from build123d import *

# Parameters (mm, degrees)
F0_W     = 36
F0_H     = 36
F1_DEPTH = 243
F3_DEPTH = 40.001


# Not quite as in the source:
# - a pattern or mirror of a feature is missing from the dataset's text; its kind, count and spacing are read off the source's solid


with BuildPart() as f1:
    # F0 (on Top) → F1 (new body, symmetric)
    with BuildSketch(Plane.XY):
        with BuildLine():
            Line((17, 20), (-17, 20))
            ThreePointArc((-17, 20), (-19.1213203436, 19.1213203436), (-20, 17))
            Line((-20, 17), (-20, -17))
            ThreePointArc((-20, -17), (-19.1213203436, -19.1213203436), (-17, -20))
            Line((-17, -20), (17, -20))
            ThreePointArc((17, -20), (19.1213203436, -19.1213203436), (20, -17))
            Line((20, -17), (20, 17))
            ThreePointArc((20, 17), (19.1213203436, 19.1213203436), (17, 20))
        make_face()
        Rectangle(F0_W, F0_H, mode=Mode.SUBTRACT)
    extrude(amount=F1_DEPTH, both=True)

    # F2 (on face) → F3 (cut, through all)
    with BuildSketch(Plane.XZ.offset(20)):
        Polygon((20, 243), (-20, 243), (20, 203), align=None)
    f3 = extrude(amount=-F3_DEPTH, mode=Mode.SUBTRACT)

    # F3_copies: F3 across plane
    add(f3.mirror(Plane(origin=(0, 0, 0), x_dir=(-1, 0, 0), z_dir=(0, 0, -1))), mode=Mode.SUBTRACT)


solid = f1.part
Design review of the part built by this model. Coordinates are the model's own, in mm. A direction names the side the tool comes from. Give positions to 0.01 mm unless a question says otherwise; leave off trailing zeros. Write each loop counter-clockwise with the first axis right and the second up, starting at its lowest first coordinate (ties: lowest second). Pieces come first, ordered by that corner, then holes. Notation, with made-up numbers: M 54.25,60.25 L 61.25,60.25 A24 cw 61.25,89.25 Z; hole C -29.5,-40 d10. An arc over 180 degrees is marked long. Answer as a JSON object with one key per item and string values. Group by question number.
1) We need section B-B (y = -13). Give the boundary of the cut face in (x, z).
2) We need section A-A (x = -9). Give the boundary of the cut face in (y, z), and give its area (3 significant figures).
3) For line 1 along X through (y, z) = (-14, -42.5), list the stretches that pass through material, from the lowest coordinate up.
4) Mouldability with a two-part tool opening along Y and no side actions: class faces 1 (the face through (0, -20, 3)), 2 (the face through (0, -19, -223)), 3 (the face through (0, -18, 3)) as released by +Y, released by -Y, zero draft, split by the parting line, or undercut.
5) Tool access review of faces 4 (the face through (0, -19, 223)), 5 (the face through (-18, 0, 3)): name each direction out of +Z, -Z, +X, -X, +Y, -Y from which nothing blocks a thin tool from reaching the whole face with its end or side.
6) We need section C-C (z = -95.5). Give the boundary of the cut face in (x, y), and give its area (3 significant figures).
Answer key:
{
 "1": {"outline": "M -20,-243 L -18,-241 L -18,241 L -20,243 Z; M 18,-205 L 20,-203 L 20,203 L 18,205 Z"},
 "2": {"outline": "M -20,-232 L -18,-232 L -18,232 L -20,232 Z; M 18,-232 L 20,-232 L 20,232 L 18,232 Z", "area": "1,860 mm²"},
 "3": {"line 1": "x = -20 to -18, 18 to 20"},
 "4": {"face 1": "released by -Y", "face 2": "zero draft", "face 3": "undercut"},
 "5": {"face 4": "+Z, +X, +Y, -Y", "face 5": "+Z, -Z"},
 "6": {"outline": "M -20,-17 A3 ccw -17,-20 L 17,-20 A3 ccw 20,-17 L 20,17 A3 ccw 17,20 L -17,20 A3 ccw -20,17 Z; hole M -18,-18 L 18,-18 L 18,18 L -18,18 Z", "area": "296 mm²"}
}
